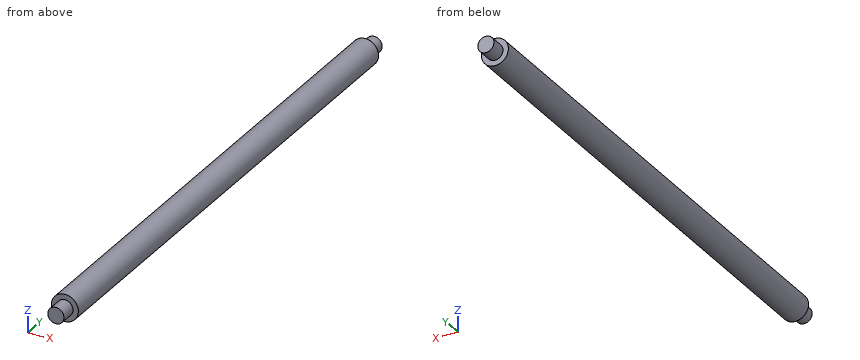
from build123d import *

# Parameters (mm, degrees)
SKETCH_1_R      = 2.5
EXTRUDE_2_DEPTH = 50
SKETCH_2_R      = 1.5
EXTRUDE_3_DEPTH = 3
EXTRUDE_START   = 3
SKETCH_3_R      = 1.5
EXTRUDE_4_DEPTH = 3


with BuildPart() as part:
    # 草图1 → 凸台-拉伸2 (new, symmetric)
    with BuildSketch(Plane(origin=(0, 0, 0), x_dir=(1, 0, 0), z_dir=(0, 1, 0))):
        with Locations(Location((0, 0, 0), (0, 0, 270))):
            Circle(SKETCH_1_R)
    extrude(amount=EXTRUDE_2_DEPTH, both=True)

    # 草图2 → 凸台-拉伸3 (add)
    with BuildSketch(Plane(origin=(0, 50, 0), x_dir=(1, 0, 0), z_dir=(0, 1, 0))):
        with Locations(Location((0, 0, 0), (0, 0, 270))):
            Circle(SKETCH_2_R)
    extrude(amount=EXTRUDE_3_DEPTH)

    # 草图3 → 凸台-拉伸4 (add)
    with BuildSketch(Plane.XZ.offset(50).offset(EXTRUDE_START)):
        with Locations(Location((0, 0, 0), (0, 0, 90))):
            Circle(SKETCH_3_R)
    extrude(amount=-EXTRUDE_4_DEPTH)


solid = part.part
Input: part model. Units: mm. Frame: model coordinates. Give positions to 0.01 mm unless a question says otherwise; leave off trailing zeros. Order: outer loops, then holes, each group sorted by start corner. A loop starts at its lowest first (then second) coordinate and runs counter-clockwise, first axis right, second up.
Q1. Section B-B on z = 0. Output: boundary loops of the cut face in (x, y), and give its area (3 significant figures).
Checked values:
outline: (-2.5, -50) - (-1.5, -50) - (-1.5, -53) - (1.5, -53) - (1.5, -50) - (2.5, -50) - (2.5, 50) - (1.5, 50) - (1.5, 53) - (-1.5, 53) - (-1.5, 50) - (-2.5, 50) - close
area: 518 mm2
Q2. Ray query, probe 1 along Y at (x, z) = (0.4, -1.7); probe 2 along Z at (x, y) = (0.3, -13.5); probe 3 along Z at (x, y) = (-2, -23.5). Return the intervals inside material, ascending.
Checked values:
probe 1: y = -50 to 50
probe 2: z = -2.48 to 2.48
probe 3: z = -1.5 to 1.5
Q3. Contact query for flat-ended pins moving along their axis: pin 1 Ø1 at (x, y) = (-1, 27) entering from -Z; pin 2 Ø1.5 at (x, y) = (-1.5, 5.5) entering from +Z. Output: stop coordinate, or through.
Checked values:
pin 1: stops at z = -2.45
pin 2: stops at z = 2.38
Q4. Section C-C on y = -43. Output: boundary loops of the cut face in (x, z).
Checked values:
outline: circle Ø5 at (0, 0)
Q5. Section A-A on x = 0. Output: boundary loops of the cut face in (y, z).
Checked values:
outline: (-53, -1.5) - (-50, -1.5) - (-50, -2.5) - (50, -2.5) - (50, -1.5) - (53, -1.5) - (53, 1.5) - (50, 1.5) - (50, 2.5) - (-50, 2.5) - (-50, 1.5) - (-53, 1.5) - close
